The listing builds one solid part. Answer for the finished solid, in the listing's coordinates (mm). A direction names the side the tool comes from. Give positions to 0.01 mm unless a question says otherwise; leave off trailing zeros. Order: outer loops, then holes, each group sorted by start corner. A loop starts at its lowest first (then second) coordinate and runs counter-clockwise, first axis right, second up. Notation, with made-up numbers: (-8, -10.75) - (23, -10.75) arc R17 cw to (23, 19.25) - close; hole circle Ø9 at (-21, 86). An arc over 180 degrees is marked (long way). Use CSV: the item, a comma, the result in double quotes.
```python
from build123d import *

# Parameters (mm, degrees)
F1_DEPTH       = 50
F4_DEPTH       = 25
F5_W           = 30
F5_H           = 60
F6_DEPTH       = 75
F8_D           = 4.4
F8_CSINK_D     = 8.96
F8_CSINK_ANGLE = 90
F9_R           = 2
F10_T1_DEPTH   = 30
F11_R          = 10
F12_SIZE       = 1.99999
F13_SIZE       = 1
F14_SIZE       = 5


# Not quite as in the source:
# - a fillet or chamfer that OpenCascade refuses, or shapes differently, is made with other operations: its cross-section is extruded or revolved along the edge and cut away or added
# - a fillet or chamfer is up to 0.001 mm smaller than in the source, because OpenCascade refuses the exact size


with BuildPart() as f1:
    # F0 (on Right) → F1 (new body)
    with BuildSketch(Plane.YZ):
        with BuildLine():
            Line((-49.4901207083, 58.9800291521), (0, 0))
            Line((0, 0), (0, 100))
            Line((0, 100), (-4, 100))
            ThreePointArc((-4, 100), (-32.2344149115, 86.0007850138), (-60.2787795686, 100.3769394581))
            Line((-60.2787795686, 100.3769394581), (-64.2787644391, 100.3879410703))
            ThreePointArc((-64.2787644391, 100.3879410703), (-60.5350609092, 78.3801837008), (-49.4901207083, 58.9800291521))
        make_face()
    extrude(amount=F1_DEPTH)

    # F3 (on offset) → F4 (cut, symmetric)
    with BuildSketch(Plane.YZ.offset(25)):
        with BuildLine():
            ThreePointArc((-32, 76), (-44.2642678148, 77.703490499), (-55.5999994652, 82.684989557))
            ThreePointArc((-55.5999994652, 82.684989557), (-49.1013266214, 68.5324924594), (-39.0785260857, 56.6132058929))
            Line((-39.0785260857, 56.6132058929), (-5, 16))
            Line((-5, 16), (-5, 76))
            Line((-5, 76), (-32, 76))
        make_face()
    extrude(amount=F4_DEPTH, both=True, mode=Mode.SUBTRACT)

    # F5 (on Top) → F6 (cut)
    with BuildSketch(Plane.XY):
        with Locations((25, -35)):
            Rectangle(F5_W, F5_H)
    extrude(amount=F6_DEPTH, mode=Mode.SUBTRACT)

    # F8 (through all)
    with Locations(Plane.XZ.offset(5)):
        with Locations((25.014353916, 63.602976501), (25.0169411302, 23.9024478942)):
            CounterSinkHole(F8_D / 2, F8_CSINK_D / 2, counter_sink_angle=F8_CSINK_ANGLE)

    # F9
    f9_edges = [f1.edges().sort_by_distance(p)[0] for p in [
        (25, -64.278764, 100.387941),
        (25, -60.27878, 100.376939),
        (25, -4, 100),
        (25, -59.21917, 75),
        (25, -55.599999, 82.68499),
        (25, -5, 76),
    ]]
    fillet(f9_edges, radius=F9_R)

    # F10: fillet of radius 2 on 1 edges, made by hand

    # F10_s2 → F10_t1 (cut)
    with BuildSketch(Plane.YZ.offset(10)):
        with BuildLine():
            ThreePointArc((-53.8387023607, 77.7281856581), (-54.0497056605, 75.8722525363), (-55.7014276886, 75))
            Line((-55.7014276886, 75), (-55.7014276886, 74.8))
            Line((-55.7014276886, 74.8), (-52.6458541761, 74.8))
            Line((-52.6458541761, 74.8), (-52.4647225466, 75.0848017263))
            ThreePointArc((-52.4647225466, 75.0848017263), (-53.6427658792, 77.7768016426), (-53.6524298279, 77.8010042239))
            Line((-53.6524298279, 77.8010042239), (-53.8387023607, 77.7281856581))
        make_face()
    extrude(amount=F10_T1_DEPTH, mode=Mode.SUBTRACT)

    # F11
    f11_edges = [f1.edges().sort_by_distance(p)[0] for p in [
        (45, -39.078526, 56.613206),
        (5, -39.078526, 56.613206),
    ]]
    fillet(f11_edges, radius=F11_R)

    # F12 (size 2 in the source; OpenCascade refuses exactly that, so slightly less here)
    f12_edges = [f1.edges().sort_by_distance(p)[0] for p in [
        (50, -32.228082, 86.000743),
        (50, -60.18128, 77.414084),
        (50, -63.689465, 99.780073),
        (50, -61.763987, 100.381024),
        (50, -60.395948, 100.173665),
        (50, -3.887164, 99.800901),
        (50, -1.508623, 100),
        (50, -24.74506, 29.490015),
    ]]
    chamfer(f12_edges, length=F12_SIZE)

    # F13
    f13_edges = [f1.edges().sort_by_distance(p)[0] for p in [
        (0, -1.508623, 100),
        (0, -3.887164, 99.800901),
        (0, -32.228082, 86.000743),
        (0, -60.395948, 100.173665),
        (0, -61.763987, 100.381024),
        (0, -63.689465, 99.780073),
        (0, -60.18128, 77.414084),
        (0, -24.74506, 29.490015),
    ]]
    chamfer(f13_edges, length=F13_SIZE)

    # F14
    f14_edges = [f1.edges().sort_by_distance(p)[0] for p in [
        (24.500005, 0, 0),
    ]]
    chamfer(f14_edges, length=F14_SIZE)


solid = f1.part
```
Item 1: Find the intervals of material crossed by line 1 along Y through (x, z) = (23, 51.5); line 2 along Z through (x, y) = (7, -24.5); line 3 along Z through (x, y) = (37, -31), in increasing order.
Taken from the geometry:
line 1,"-5 to 0"
line 2,"29.2 to 39.24, 76 to 86.81"
line 3,"76 to 86.01"
Item 2: Which of the six approach directions +Z, -Z, +X, -X, +Y, -Y give full straight-line access (tool end or side, diameter ignored) to faces 4 (the face through (25, -57, 75)), 5 (the face through (27.215, -1.341, 23.999)), 6 (the face through (49, -1, 99)), 7 (the face through (24.65, -5.6, 75.43)), 8 (the face through (25.32, -2.83, 65.89))?
Taken from the geometry:
face 4,"-Z, -Y"
face 5,"+Y, -Y"
face 6,"+Z, +X, +Y"
face 7,"+X, -X"
face 8,"-Y"
Item 3: Each of these flat-tipped pins is pushed along its axis until it touches: pin 1 (8 mm diameter, centred on x = 15, z = 16, fed in from -Y); pin 2 (12 mm diameter, centred on x = 16.5, y = -30, fed in from +Z); pin 3 (0.7 mm diameter, centred on x = 29, y = -56.5, fed in from -Z). Where does it stop, or does it pass through?
Taken from the geometry:
pin 1,"y = -5"
pin 2,"z = 86.93"
pin 3,"z = 75"
Item 4: The part is cut by section B-B (y = -36). Count the separate pieces of the cut face and the enclosed holes in it, and give its area (3 significant figures).
Taken from the geometry:
separate pieces,"3"
enclosed holes,"0"
area,"697 mm^2"
Item 5: The part is cut by section A-A (z = 54). Give the vertices of the cut face in (x, y), and give its area (3 significant figures).
Taken from the geometry:
outline,"(0, -44.01) - (1, -45.31) - (10, -45.31) - (10, -36.89) - (0, -36.89) - close; (0, -5) - (50, -5) - (50, 0) - (0, 0) - close; (40, -45.31) - (48, -45.31) - (50, -42.7) - (50, -36.89) - (40, -36.89) - close"
area,"415 mm^2"
Item 6: The mould has two halves that part along Z. Classify faces 1 (the face through (25, -5, 40)), 2 (the face through (10, -32, 42)), 3 (the face through (24, -1, 100)): +Z half, -Z half, draft (parallel to the pull), parting line (faces both ways), or undercut.
Taken from the geometry:
face 1,"undercut"
face 2,"draft"
face 3,"+Z half"
